Can you work these out from the model? Positions are in its coordinate system, mm. Face numbers are marked on the shaded views. A direction names the side the tool comes from. Give positions to 0.01 mm unless a question says otherwise; leave off trailing zeros. Loops run counter-clockwise (first coordinate to the right, second up) from the corner with the lowest first, then second, coordinate; pieces in that order, holes last.
from build123d import *

# Parameters (mm, degrees)
SKETCH1_W                       = 42.960806382
SKETCH1_H                       = 31.115
BOSS_EXTRUDE1_DEPTH             = 12.7
SKETCH2_W                       = 42.960806382
SKETCH2_H                       = 22.225
BOSS_EXTRUDE2_DEPTH             = 19.05
BOSS_EXTRUDE3_DEPTH             = 22.225
DRAFT1_START                    = 15
DRAFT1_OUTLINE_W                = 22.225
DRAFT1_OUTLINE_H                = 19.270002336
DRAFT1_DEPTH                    = 6.752762537
BOSS_EXTRUDE4_REACH             = 69.308
SKETCH6_W                       = 42.960806382
SKETCH6_H                       = 4.445
DRAFT3_ANGLE                    = 20
DRAFT4_ANGLE                    = 20
BOSS_EXTRUDE5_DEPTH             = 22.225
F_6_CLEARANCE_HOLE1_D           = 4.3053
F_6_CLEARANCE_HOLE2_D           = 4.3053
F_6_CLEARANCE_HOLE2_ON_FACE_2_D = 4.3053
HOLE1_AT_2_COUNT                = 2
HOLE1_AT_2_PITCH                = 10.16
HOLE2_AT_2_COUNT                = 2
HOLE2_AT_2_PITCH                = 10.16
CUT_EXTRUDE1_DEPTH              = 70.758470007
CHAMFER1_SIZE                   = 2.54
CHAMFER2_SIZE                   = 0.762
HOLE3_AT_2_COUNT                = 2
HOLE3_AT_2_PITCH                = 19.49777111
HOLE3_AT_3_COUNT                = 2
HOLE3_AT_3_PITCH                = 29.565413971
HOLE4_AT_2_COUNT                = 2
HOLE4_AT_2_PITCH                = 22.225
HOLE4_AT_3_COUNT                = 2
HOLE4_AT_3_PITCH                = 29.565413971


with BuildPart() as part:
    # Sketch1 → Boss-Extrude1 (new body)
    with BuildSketch(Plane.XY):
        with Locations((1.668403191, -9.5885)):
            Rectangle(SKETCH1_W, SKETCH1_H)
    extrude(amount=BOSS_EXTRUDE1_DEPTH)

    # Sketch2 → Boss-Extrude2 (add)
    with BuildSketch(Plane.XY.offset(12.7)):
        with Locations((1.668403191, -9.5885)):
            Rectangle(SKETCH2_W, SKETCH2_H)
    extrude(amount=BOSS_EXTRUDE2_DEPTH)

    # Sketch3 → Boss-Extrude3 (add)
    with BuildSketch(Plane.XZ.offset(20.701)):
        Polygon((23.148806382, 31.75), (53.759077492, 31.75), (53.759077492, 0), (44.234077492, 0), (44.234077492, 18.107878998), (23.148806382, 18.107878998), align=None)
    extrude(amount=-BOSS_EXTRUDE3_DEPTH)

    # Draft1: read off the stored shape, not the designer's step
    # Draft1 outline → Draft1 (add)
    with BuildSketch(Plane(origin=(0, 0, 0), x_dir=(0, 1, 0), z_dir=(0.9396926207859083, 0, -0.3420201433256691)).offset(DRAFT1_START)):
        with Locations((-9.5885, 17.552359245)):
            Rectangle(DRAFT1_OUTLINE_W, DRAFT1_OUTLINE_H)
    extrude(amount=DRAFT1_DEPTH)

    # Sketch6 → Boss-Extrude4 (add, up to next)
    with BuildSketch(Plane.XY.offset(31.75), mode=Mode.PRIVATE) as boss_extrude4_sk1:
        with Locations((1.668403191, 3.7465)):
            Rectangle(SKETCH6_W, SKETCH6_H)
    boss_extrude4_tool1 = extrude(boss_extrude4_sk1.sketch, amount=-BOSS_EXTRUDE4_REACH, mode=Mode.PRIVATE) - part.part
    # Sketch6 → Boss-Extrude4 (add, up to next)
    with BuildSketch(Plane.XY.offset(31.75), mode=Mode.PRIVATE) as boss_extrude4_sk2:
        with Locations((1.668403191, -22.9235)):
            Rectangle(SKETCH6_W, SKETCH6_H)
    boss_extrude4_tool2 = extrude(boss_extrude4_sk2.sketch, amount=-BOSS_EXTRUDE4_REACH, mode=Mode.PRIVATE) - part.part
    add(boss_extrude4_tool1.solids().sort_by_distance((1.668403, 3.7465, 31.75))[0])
    add(boss_extrude4_tool2.solids().sort_by_distance((1.668403, -22.9235, 31.75))[0])

    # Draft3
    draft3_faces = [part.faces().sort_by_distance(p)[0] for p in [
        (23.148806382, -22.9235, 15.875),
    ]]
    draft(draft3_faces, Plane(origin=(23.148806382, -20.701, 31.75), x_dir=(-1, 0, 0), z_dir=(0, -1, 0)), DRAFT3_ANGLE)

    # Draft4
    draft4_faces = [part.faces().sort_by_distance(p)[0] for p in [
        (23.148806382, 3.7465, 15.875),
    ]]
    draft(draft4_faces, Plane(origin=(23.148806382, 1.524, 31.75), x_dir=(1, 0, 0), z_dir=(0, 1, 0)), DRAFT4_ANGLE)

    # Sketch8 → Boss-Extrude5 (add)
    with BuildSketch(Plane.XZ.offset(20.701)):
        Polygon((29.739535343, 18.107878998), (23.148806382, 0), (44.234077492, 0), (44.234077492, 18.107878998), align=None)
    extrude(amount=-BOSS_EXTRUDE5_DEPTH)

    # #6 Clearance Hole1 (through all)
    with Locations(Plane(origin=(0, -20.701, 0), x_dir=(-1, 0, 0), z_dir=(0, -1, 0))):
        with Locations((-48.996577492, -26.9875), (-48.996577492, -4.7625), (-29.498806382, -26.9875)):
            Hole(F_6_CLEARANCE_HOLE1_D / 2)

    # #6 Clearance Hole2 (through all)
    with Locations(Plane(origin=(-14.986, -25.146, 3.81), x_dir=(-1, 0, 0), z_dir=(0, -1, 0))):
        with Locations((0, 0), (-10.16, 0)):
            Hole(F_6_CLEARANCE_HOLE2_D / 2)

    # #6 Clearance Hole2 on face 2 (through all)
    with Locations(Plane(origin=(14.986, 5.969, 3.81), x_dir=(0, 0, 1), z_dir=(0, 1, 0))):
        with Locations((0, 0), (0, -10.16)):
            Hole(F_6_CLEARANCE_HOLE2_ON_FACE_2_D / 2)

    # Sketch18 → Hole1 (revolve, cut)
    with BuildSketch(Plane(origin=(-4.826, 5.969, 3.81), x_dir=(0, 0, 1), z_dir=(1, 0, 0))):
        Polygon((0, 0), (0, 3.81), (2.5273, 3.81), (2.6543, 0), align=None)
    hole1 = revolve(axis=Axis((-4.826, -104.031, 3.81), (0, 1, 0)), mode=Mode.SUBTRACT)

    # Hole1 at 2: Hole1 ×2
    with Locations(*[(-i * HOLE1_AT_2_PITCH, 0, 0) for i in range(1, HOLE1_AT_2_COUNT)]):
        add(hole1, mode=Mode.SUBTRACT)

    # Sketch20 → Hole2 (revolve, cut)
    with BuildSketch(Plane(origin=(4.826, -25.146, 3.81), x_dir=(0, 0, -1), z_dir=(1, 0, 0))):
        Polygon((0, 0), (0, 3.81), (2.5273, 3.81), (2.6543, 0), align=None)
    hole2 = revolve(axis=Axis((4.826, 84.854, 3.81), (0, -1, 0)), mode=Mode.SUBTRACT)

    # Hole2 at 2: Hole2 ×2
    with Locations(*[(i * HOLE2_AT_2_PITCH, 0, 0) for i in range(1, HOLE2_AT_2_COUNT)]):
        add(hole2, mode=Mode.SUBTRACT)

    # Sketch21 → Cut-Extrude1 (cut, through all)
    with BuildSketch(Plane(origin=(0, 5.969, 0), x_dir=(1, 0, 0), z_dir=(0, 1, 0))):
        Polygon((-19.812, -9.525), (-19.812, -31.75), (15.180958691, -31.75), align=None)
    extrude(amount=-CUT_EXTRUDE1_DEPTH, mode=Mode.SUBTRACT)

    # Chamfer1
    chamfer1_edges = [part.edges().sort_by_distance(p)[0] for p in [
        (53.759077492, -9.5885, 31.75),
        (53.759077492, -9.5885, 0),
    ]]
    chamfer(chamfer1_edges, length=CHAMFER1_SIZE)

    # Chamfer2
    chamfer2_edges = [part.edges().sort_by_distance(p)[0] for p in [
        (-19.812, -25.146, 4.7625),
        (-19.812, 5.969, 4.7625),
        (0.859479345, -25.146, 0),
        (-19.812, -9.5885, 0),
        (0.859479345, 5.969, 0),
    ]]
    chamfer(chamfer2_edges, length=CHAMFER2_SIZE)

    # Sketch23 → Hole3 (revolve, cut)
    with BuildSketch(Plane(origin=(29.498806382, 1.524, 26.9875), x_dir=(0, 0, 1), z_dir=(1, 0, 0))):
        Polygon((0, 0), (0, 3.81), (2.5781, 3.81), (2.7813, 0), align=None)
    hole3 = revolve(axis=Axis((29.498806382, -108.476, 26.9875), (0, 1, 0)), mode=Mode.SUBTRACT)

    # Hole3 at 2: Hole3 ×2
    with Locations(*[(i * HOLE3_AT_2_PITCH, 0, 0) for i in range(1, HOLE3_AT_2_COUNT)]):
        add(hole3, mode=Mode.SUBTRACT)

    # Hole3 at 3: Hole3 ×2
    with Locations(*[Vector(0.6594790497158223, 0, -0.7517229429689612) * (i * HOLE3_AT_3_PITCH) for i in range(1, HOLE3_AT_3_COUNT)]):
        add(hole3, mode=Mode.SUBTRACT)

    # Sketch25 → Hole4 (revolve, cut)
    with BuildSketch(Plane(origin=(48.996577492, -20.701, 4.7625), x_dir=(0, 0, -1), z_dir=(1, 0, 0))):
        Polygon((0, 0), (0, 3.81), (2.5781, 3.81), (2.7813, 0), align=None)
    hole4 = revolve(axis=Axis((48.996577492, 89.299, 4.7625), (0, -1, 0)), mode=Mode.SUBTRACT)

    # Hole4 at 2: Hole4 ×2
    with Locations(*[(0, 0, i * HOLE4_AT_2_PITCH) for i in range(1, HOLE4_AT_2_COUNT)]):
        add(hole4, mode=Mode.SUBTRACT)

    # Hole4 at 3: Hole4 ×2
    with Locations(*[Vector(-0.6594790497158223, 0, 0.7517229429689612) * (i * HOLE4_AT_3_PITCH) for i in range(1, HOLE4_AT_3_COUNT)]):
        add(hole4, mode=Mode.SUBTRACT)


solid = part.part
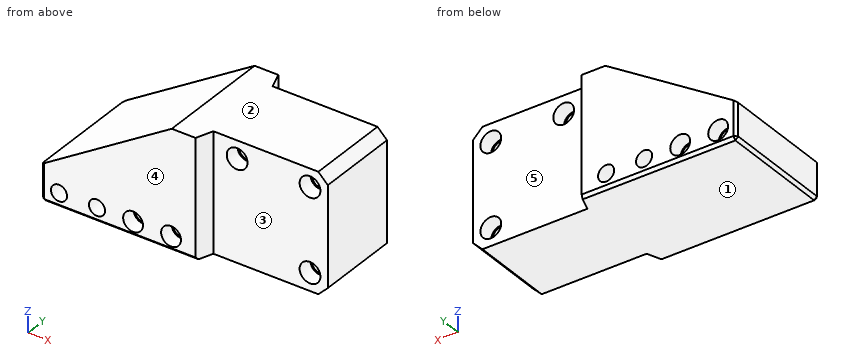
(1) Suppose I cut it at A-A on y = -4. Give the number of separate pieces and of enclosed holes in the cut face, plus the area to 3 significant figures.
Returned:
separate pieces: 1
enclosed holes: 7
area: 1,840 mm2
(2) Please list where these lines run through material, in increasing order: probe 1 along X at (y, z) = (-17, 3); probe 2 along Y at (x, z) = (26, 7); probe 3 along X at (y, z) = (-20.5, 24.5).
Returned:
probe 1: x = -19.81 to -16.98, -12.99 to -6.82, -2.83 to 2.83, 6.82 to 12.99, 16.98 to 47.11, 50.89 to 53.76
probe 2: y = -20.7 to 1.52
probe 3: x = 3.77 to 28.28, 30.72 to 47.78, 50.22 to 53.76
(3) Suppose I cut it at D-D on x = -10. List the corners of the cut face in (y, z) for me.
Returned:
outline: (-25.15, 0.76) - (-24.38, 0) - (5.21, 0) - (5.97, 0.76) - (5.97, 15.76) - (-25.15, 15.76) - close
(4) Suppose I cut it at B-B on y = 4. List the corners of the cut face in (x, z) for me (3 decimals).
Returned:
outline: (-19.812, 0.762) - (-19.05, 0) - (22.248, 0) - (22.248, 31.75) - (15.181, 31.75) - (-19.812, 9.525) - close; hole circle Ø5.177 at (-14.986, 3.81); hole circle Ø5.177 at (-4.826, 3.81); hole circle Ø4.305 at (4.826, 3.81); hole circle Ø4.305 at (14.986, 3.81)
(5) Suppose I cut it at C-C on z = 12. List the corners of the cut face in (x, y) for me.
Returned:
outline: (-15.92, -25.15) - (21.53, -25.15) - (23.15, -20.7) - (53.76, -20.7) - (53.76, 1.52) - (23.15, 1.52) - (21.53, 5.97) - (-15.92, 5.97) - close
(6) Thinking about a two-plate mould opening in Z: for the marked faces 1, 2 and 3, which applies, pulls with the +Z half, pulls with the -Z half, needs draft (parallel to the pull), parting line crosses it, or undercut?
Returned:
face 1: pulls with the -Z half
face 2: pulls with the +Z half
face 3: needs draft
(7) Will these pins go through, and if not, where does the flat tip stop? P1, Ø4, axis at x = -4.826, z = 3.81, coming from the -Y side; P2, Ø15.5, axis at x = 34, z = 11, coming from the -Y side; P3, Ø10, axis at x = 35.5, z = 22, coming from the +Y side; P4, Ø4, axis at x = 49, z = 4.5, coming from the -Y side.
Returned:
P1: passes through
P2: stops at y = -20.7
P3: stops at y = 1.52
P4: stops at y = -16.89
(8) Which directions (+Z, -Z, +X, -X, +Y, -Y) give clear straight access to the entire face, cutting with the end or side of a thin tool? Please do the marked faces 4 and 5.
Returned:
face 4: +Z, -Z, +X, -X, -Y
face 5: +Z, -Z, +X, +Y
